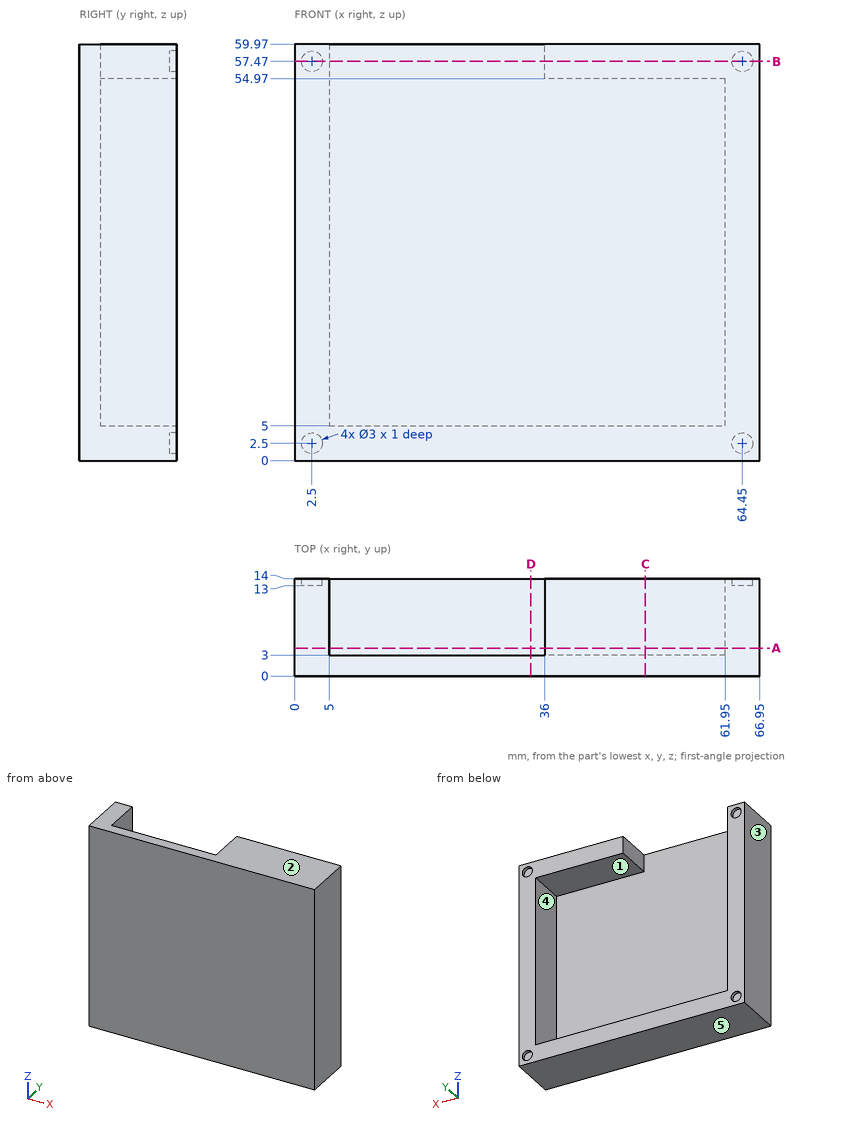
Input: dimensioned drawing with shaded views. Units: mm. Origin: part minimum x, y, z. A direction names the side the tool comes from. Give positions to 0.01 mm unless a question says otherwise; leave off trailing zeros. Write each loop counter-clockwise with the first axis right and the second up, starting at its lowest first coordinate (ties: lowest second). Pieces come first, ordered by that corner, then holes.
Q1. Section A-A, the plane y = 4. Output: boundary loops of the cut face in (x, z), plus the area to 3 significant figures.
Q2. Section C-C, the plane x = 50.5. Output: boundary loops of the cut face in (y, z).
Q3. Pull-direction query (Z, two-part tool) for the marked faces 3, 4 and 5; classes: pulls with the +Z half, pulls with the -Z half, needs draft (parallel to the pull), parting line crosses it, or undercut.
Q4. Section B-B, the plane z = 57.47. Output: boundary loops of the cut face in (x, y).
Q5. Material intervals for probe 1 along X at (y, z) = (13.6, 2.5); probe 2 along Z at (x, y) = (64.45, 13.6); probe 3 along X at (y, z) = (13.3, 57.47), sorted ascending.
Q6. Section D-D, the plane x = 34. Output: boundary loops of the cut face in (y, z).
Q7. First-contact query: P1, Ø1.5, axis at x = 65, z = 57.5, coming from the +Y side; P2, Ø3, axis at x = 48, z = 40, coming from the +Y side; P3, Ø3, axis at x = 18.5, y = 8.5, coming from the +Z side. Flat tips, straight axial feed; report the tip coordinate or a pass-through.
Q8. Set-up query: the marked faces 1 and 2. Return all of +Z, -Z, +X, -X, +Y, -Y with unobstructed straight access to the full face (end or side cutting, diameter ignored); none if empty.
Filled in:
1. outline: (0, 0) - (66.95, 0) - (66.95, 59.97) - (36, 59.97) - (36, 54.97) - (61.95, 54.97) - (61.95, 5) - (5, 5) - (5, 59.97) - (0, 59.97) - close
1. area: 1,010 mm2
2. outline: (0, 0) - (14, 0) - (14, 5) - (3, 5) - (3, 54.97) - (14, 54.97) - (14, 59.97) - (0, 59.97) - close
3. face 3: needs draft
3. face 4: undercut
3. face 5: pulls with the -Z half
4. outline: (0, 0) - (66.95, 0) - (66.95, 14) - (65.95, 14) - (65.95, 13) - (62.95, 13) - (62.95, 14) - (36, 14) - (36, 3) - (5, 3) - (5, 14) - (4, 14) - (4, 13) - (1, 13) - (1, 14) - (0, 14) - close
5. probe 1: x = 0 to 1, 4 to 62.95, 65.95 to 66.95
5. probe 2: z = 0 to 1, 4 to 55.97, 58.97 to 59.97
5. probe 3: x = 0 to 1, 4 to 5, 36 to 62.95, 65.95 to 66.95
6. outline: (0, 0) - (14, 0) - (14, 5) - (3, 5) - (3, 59.97) - (0, 59.97) - close
7. P1: stops at y = 13
7. P2: stops at y = 3
7. P3: stops at z = 5
8. face 1: +Y
8. face 2: +Z, +X, -X, +Y, -Y
